Work out the finished part from the listing and answer in its coordinate system (mm). A direction names the side the tool comes from. Round coordinates to 2 decimals unless told otherwise and drop trailing zeros. Loops run counter-clockwise (first coordinate to the right, second up) from the corner with the lowest first, then second, coordinate; pieces in that order, holes last. Notation, with made-up numbers: (2, 86) - (54, 86) arc R6 cw to (54, 90) - close; hole circle Ø5 at (-8.5, 36). An arc over 180 degrees is marked (long way). Answer as CSV lines item,"result". Start each with the question number.
Q1. Section A-A on z = 6 is taken. Write down the section's boundary in (x, y).
Q2. For faces 1 (the face through (-10.6, 9, 5)), 2 (the face through (9.763, 5.824, 3.451)), 3 (the face through (-11.5, 0, 5)), determine the directions among +Z, -Z, +X, -X, +Y, -Y from which every point of the face is accessible in a straight line to the end or side of a thin tool.
Q3. Straight lines are drawn through the part: L1, parallel to Y at x = -10.5, z = 5; L2, parallel to Y at x = -2.5, z = 2.5; L3, parallel to X at y = 7, z = 0.75. For each, find the intervals that lie inside material, in ascending order. Write a range as [from, to].
Q4. Each of these flat-tipped pins is pushed along its axis until it touches: pin 1 Ø1.5 at (x, y) = (8, 2.5) entering from +Z; pin 2 Ø3 at (y, z) = (-2, 5.5) entering from -X; pin 3 Ø1 at (y, z) = (-5.5, 4.5) entering from +X; pin 4 Ø1.6 at (x, z) = (-10.5, 5) entering from -Y. Where does it stop, or does it pass through?
Q5. Section D-D on z = 0.5 is taken. Write down the section's boundary in (x, y).
Q6. Section B-B on x = 9 is taken. Write down the section's boundary in (y, z), then the cut area to 3 significant figures.
Q7. Section C-C on y = 6.5 is taken. Write down the section's boundary in (x, z), then the cut area to 3 significant figures.
Q8. The mould has two halves that part along X. Classify faces 4 (the face through (15, 0, 1)), 5 (the face through (11, -4.378, 5)), 6 (the face through (3, 0, 1.5)): +X half, -X half, draft (parallel to the pull), parting line (faces both ways), or undercut.
Autodesk Fusion 360 part; units mm, degrees
sketch "Schizzo1" plane through (0, 0, 0) normal (0, 0, 1) x (1, 0, 0)
  line L0 (15, -11) -> (-15, -11)
  line L1 (-15, -11) -> (-15, 11)
  line L2 (-15, 11) -> (15, 11)
  line L3 (15, 11) -> (15, -11)
  line L4 (15, -11) -> (-15, 11) construction
  line L5 (-15, -11) -> (15, 11) construction
  circle A0 centre (-10.5, 6.5) radius 1
  line L6 (0, 0) -> (0, 29.5876)
  circle A1 centre (10.5, 6.5) radius 1
  line L7 (-4.5, -3) -> (-9.5, -3)
  line L8 (-9.5, -3) -> (-9.5, 3)
  line L9 (-9.5, 3) -> (-4.5, 3)
  line L10 (-4.5, 3) -> (-4.5, -3)
  line L11 (-4.5, -3) -> (-9.5, 3) construction
  line L12 (-9.5, -3) -> (-4.5, 3) construction
  line L13 (4.5, -3) -> (9.5, -3)
  line L14 (9.5, -3) -> (9.5, 3)
  line L15 (9.5, 3) -> (4.5, 3)
  line L16 (4.5, 3) -> (4.5, -3)
  circle A2 centre (-10.5, 6.5) radius 2.5
  circle A3 centre (10.5, 6.5) radius 2.5
  line L17 (-9.5, 4.3778) -> (-11.5, 4.3778)
  line L18 (-11.5, 4.3778) -> (-11.5, -4.3778)
  line L19 (-11.5, -4.3778) -> (-9.5, -4.3778)
  line L20 (-9.5, -4.3778) -> (-9.5, 4.3778)
  line L21 (-9.5, 4.3778) -> (-11.5, -4.3778) construction
  line L22 (-11.5, 4.3778) -> (-9.5, -4.3778) construction
  line L23 (9.5, 4.3778) -> (11.5, 4.3778)
  line L24 (11.5, -4.3778) -> (9.5, -4.3778)
  line L25 (11.5, 4.3778) -> (11.5, -4.3778)
  line L26 (9.5, -3) -> (9.5, 3)
  line L27 (9.5, -4.3778) -> (9.5, 4.3778)
  point P0 (-7, 0)
  point P1 (-10.5, 0)
  dimension "d1" = 30
  dimension "d2" = 22
  dimension "d3" = 2
  dimension "d4" = 10.5
  dimension "d6" = 4.5
  dimension "d7" = 4.5
  dimension "d8" = 5
  dimension "d9" = 6
  dimension "d10" = 5
  dimension "d11" = 5
  dimension "d12" = 2
  dimension "d13" = 8.7557
  dimension "d14" = 10.5
extrude "Estrusione1" add sketch "Schizzo1" along normal blind 3 contours L0 L1 L2 L3 | L8 A2 L18 L19 L20 | A2 L17 L18 L20 | A2 L17 L18 L20 | L14 A3 L24 L25 L26 L27 | A3 L23 L25 L27 | A3 L23 L25 L27
extrude "Estrusione2" add sketch "Schizzo1" along normal blind 4 from surface at 3 contours L8 A2 L18 L19 L20 | A2 L17 L18 L20 | A2 L17 L18 L20 | L14 A3 L24 L25 L26 L27 | A3 L23 L25 L27 | A3 L23 L25 L27
chamfer "Smusso1" distance 3 angle 45 2 edges at (-4.5, 0, 3) (4.5, 0, 3)
equation "d4 = ( 21 / 2 ) * 1 mm"
equation "d14 = ( 21 / 2 ) * 1 mm"
Findings:
1,outline,"(-11.5, -4.38) - (-9.5, -4.38) - (-9.5, 4.21) arc R2.5 ccw (long way) to (-11.5, 4.21) - close; (9.5, -4.38) - (11.5, -4.38) - (11.5, 4.21) arc R2.5 ccw (long way) to (9.5, 4.21) - close; hole circle Ø2 at (-10.5, 6.5); hole circle Ø2 at (10.5, 6.5)"
2,face 1,"+Z"
2,face 2,"+Z, -Z"
2,face 3,"+Z, -X, -Y"
3,L1,"y = [-4.38, 5.5], [7.5, 9]"
3,L2,"y = [-11, -3], [3, 11]"
3,L3,"x = [-15, -11.37], [-9.63, 9.63], [11.37, 15]"
4,pin 1,"stops at z = 3"
4,pin 2,"stops at x = -11.5"
4,pin 3,"passes through"
4,pin 4,"stops at y = -4.38"
5,outline,"(-15, -11) - (15, -11) - (15, 11) - (-15, 11) - close; hole circle Ø2 at (-10.5, 6.5); hole (-9.5, -3) - (-4, -3) - (-4, 3) - (-9.5, 3) - close; hole (4, -3) - (9.5, -3) - (9.5, 3) - (4, 3) - close; hole circle Ø2 at (10.5, 6.5)"
6,outline,"(-11, 0) - (-3, 0) - (-3, 3) - (-11, 3) - close; (3, 0) - (11, 0) - (11, 3) - (8.5, 3) - (8.5, 7) - (4.5, 7) - (4.5, 3) - (3, 3) - close"
6,area,"64.0 mm^2"
7,outline,"(-15, 0) - (-11.5, 0) - (-11.5, 7) - (-13, 7) - (-13, 3) - (-15, 3) - close; (-9.5, 0) - (9.5, 0) - (9.5, 7) - (8, 7) - (8, 3) - (-8, 3) - (-8, 7) - (-9.5, 7) - close; (11.5, 0) - (15, 0) - (15, 3) - (13, 3) - (13, 7) - (11.5, 7) - close"
7,area,"102 mm^2"
8,face 4,"+X half"
8,face 5,"draft"
8,face 6,"undercut"
